from build123d import *

# Parameters (mm, degrees)
BOSS_EXTRUDE3_DEPTH = 1.5875
FILLET1_R           = 6.35


with BuildPart() as part:
    # Sketch3 → Boss-Extrude3 (new body, symmetric)
    with BuildSketch(Plane(origin=(0, 0, 0), x_dir=(1, 0, 0), z_dir=(0, 1, 0))):
        Polygon((-77.47, -25.4), (-77.47, -101.9175), (-25.4, -101.9175), (-25.4, -100.33), (-4, -100.33), (-4, -97.33), (4, -97.33), (4, -100.33), (25.4, -100.33), (25.4, -101.9175), (77.47, -101.9175), (77.47, -25.4), (59.182, -25.4), (59.182, 25.4), (77.47, 25.4), (77.47, 101.9175), (25.4, 101.9175), (25.4, 100.33), (4, 100.33), (4, 97.33), (-4, 97.33), (-4, 100.33), (-25.4, 100.33), (-25.4, 101.9175), (-77.47, 101.9175), (-77.47, 25.4), (-59.182, 25.4), (-59.182, -25.4), align=None)
    extrude(amount=BOSS_EXTRUDE3_DEPTH, both=True)

    # Fillet1
    fillet1_edges = [part.edges().sort_by_distance(p)[0] for p in [
        (-77.47, 0, -101.9175),
        (77.47, 0, -101.9175),
        (77.47, 0, -25.4),
        (59.182, 0, -25.4),
        (59.182, 0, 25.4),
        (77.47, 0, 25.4),
        (77.47, 0, 101.9175),
        (-77.47, 0, 101.9175),
        (-77.47, 0, 25.4),
        (-59.182, 0, 25.4),
        (-59.182, 0, -25.4),
        (-77.47, 0, -25.4),
    ]]
    fillet(fillet1_edges, radius=FILLET1_R)


solid = part.part
Verification items for the finished model (mm, model axes). A direction names the side the tool comes from. Give positions to 0.01 mm unless a question says otherwise; leave off trailing zeros. Loops run counter-clockwise (first coordinate to the right, second up) from the corner with the lowest first, then second, coordinate; pieces in that order, holes last. Notation, with made-up numbers: (86, 79) - (99, 79) arc R21 cw to (99, 106) - close; hole circle Ø5 at (8.25, 9.5). An arc over 180 degrees is marked (long way). Write item = value, one per line. Start each with the question number.
Q1. Cross-section at A-A, the plane z = -11.5. Enter the section's corners in (x, y).
Q2. Tool access check on faces 4 (the face through (75.66, 0.02, -27.31)), 5 (the face through (-61, 0, -23.5)), 6 (the face through (-75.66, 0.02, -100.01)). Record the directions out of +Z, -Z, +X, -X, +Y, -Y that give a thin tool (end or side, any length) a straight path to the whole face; none if there is none.
Q3. Thickness scan on line 1 (X direction, y = -1.3, z = 1); line 2 (Z direction, x = 24, y = 0.35); line 3 (Z direction, x = -62.5, y = 0.1). Record the ranges inside material, lowest first.
Q4. Depth check by flat-ended pin: P1, Ø1, axis at x = 10.5, y = -0.5, coming from the +Z side; P2, Ø0.5, axis at y = -0.5, z = 101, coming from the +X side; P3, Ø1.5, axis at y = 0.5, z = 99, coming from the -X side. Enter the tip coordinate at first touch or a pass-through.
Q5. Mould release check, pull along Z, two halves, no side actions. Record for faces 1 (the face through (-75.66, 0.02, 100.01)), 2 (the face through (-1, -1.588, -1)), 3 (the face through (75.56, 0.02, 27.21)): released by +Z, released by -Z, zero draft, split by the parting line, or undercut.
Q6. Cross-section at B-B, the plane x = -13. Enter the section's corners in (y, z), and give its area (3 significant figures).
Answer key:
q1.outline = (-59.18, -1.59) - (59.18, -1.59) - (59.18, 1.59) - (-59.18, 1.59) - close
q2.face_4 = +X, +Y, -Y
q2.face_5 = -X, +Y, -Y
q2.face_6 = -Z, -X, +Y, -Y
q3.line_1 = -59.18 to 59.18
q3.line_2 = -100.33 to 100.33
q3.line_3 = -101.92 to -24.63, 24.63 to 101.92
q4.P1 = 100.33
q4.P2 = 74.79
q4.P3 = -76.88
q5.face_1 = released by +Z
q5.face_2 = zero draft
q5.face_3 = undercut
q6.outline = (-1.59, -100.33) - (1.59, -100.33) - (1.59, 100.33) - (-1.59, 100.33) - close
q6.area = 637 mm^2
